Read the model definition and answer for the solid it produces. Units are mm, in the model's axes. A direction names the side the tool comes from. Give positions to 0.01 mm unless a question says otherwise; leave off trailing zeros. Order: outer loops, then holes, each group sorted by start corner. A loop starts at its lowest first (then second) coordinate and runs counter-clockwise, first axis right, second up. Notation, with made-up numbers: (20, -38.5) - (45, -38.5) arc R17 ccw to (45, -26.5) - close; hole circle Ø11 at (-33, 75.25). An arc over 180 degrees is marked (long way). Use a Markdown table: item, result. Add a question column.
1. For a pull along Z with two mould halves and no side action, classify faces 1 (the flat face through (33, 14, 40)), 2 (the cylindrical face through (124.91, 3.17, 0.9)), 3 (the flat face through (-2, 65, 22)), 4 (the cylindrical face through (-124.91, 3.17, 44.1)) as released by +Z, released by -Z, zero draft, split by the parting line, or undercut.
2. A cutting plane is placed at A-A on x = -21. Determine the outline of the cut face in (y, z).
3. Consider L1, parallel to Z at x = 17, y = -53; L2, parallel to Y at x = 48, z = 32; L3, parallel to X at y = 0, z = 3. Determine where each line is inside the solid, lowest interval first.
4. A cutting plane is placed at B-B on z = 31.5. Determine the outline of the cut face in (x, y).
5. A flat-ended cylindrical pin translates along its axis: P1, Ø17.5, axis at x = 11.5, z = 15, coming from the -Y side. Find the tip coordinate at first contact, or state that the pin passes through.
6. A cutting plane is placed at C-C on y = -21. State how many separate pieces and enclosed holes the cut face has, and give its area (3 significant figures).
7. Which of the six approach directions +Z, -Z, +X, -X, +Y, -Y give full straight-line access (tool end or side, diameter ignored) to faces 5 (the flat face through (-33, 18, 0)), 6 (the flat face through (33, 14, 5))?
Autodesk Inventor part; units mm, degrees
ref_plane "Work Plane2" through (142.5, 0, 0) normal (1, 0, 0) x (0, 1, 0)
ref_plane "Work Plane3" through (140, 0, 0) normal (1, 0, 0) x (0, 1, 0)
ref_plane "XZ Plane" through (0, 0, 0) normal (0, 1, 0) x (-1, 0, 0)
sketch "Sketch1" plane through (0, 0, 0) normal (0, 0, 1) x (1, 0, 0)
  circle A0 centre (0, 0) radius 35
  line L0 (0, 0) -> (0, 35)
  line L1 (0, 0) -> (0, -35)
  line L2 (110, -60) -> (141.25, 65)
  line L3 (-110, -60) -> (-141.25, 65)
  line L4 (0, -35) -> (0, -60)
  line L5 (0, -60) -> (110, -60)
  line L6 (0, -60) -> (-110, -60)
  line L7 (0, 35) -> (0, 65)
  line L8 (0, 65) -> (141.25, 65)
  line L9 (0, 65) -> (-141.25, 65)
extrude "Extrusion3" add sketch "Sketch1" along normal blind 45 contours A0 L7 L8 L2 L5 L4 | A0 L4 L6 L3 L9 L7
ref_plane "Work Plane2" through (142.5, 0, 0) normal (1, 0, 0) x (0, 1, 0)
fillet "Fillet2" radius 3 8 edges at (-141.25, 65, 22.5) (141.25, 65, 22.5) (125.625, 2.5, 45) (-125.625, 2.5, 45) (-125.625, 2.5, 0) (125.625, 2.5, 0) (0, -60, 0) (0, -60, 45)
sketch "Sketch5" plane through (142.5, 0, 0) normal (1, 0, 0) x (0, 1, 0)
  point P0 (0, 0)
ref_plane "Work Plane3" through (140, 0, 0) normal (1, 0, 0) x (0, 1, 0)
sketch "Sketch6" plane through (140, 0, 0) normal (1, 0, 0) x (0, 1, 0)
  line L0 (-56.5599, 40) -> (60, 40)
  line L1 (60, 40) -> (60, 5)
  line L2 (60, 5) -> (-60.1868, 5)
  line L3 (-56.5599, 40) -> (60, 5) construction
  line L4 (60, 40) -> (-60.1868, 5) construction
  line L5 (65, 0) -> (65, 45)
  line L6 (-56.5599, 40) -> (-64.3318, 40)
  line L7 (-64.3318, 40) -> (-64.3318, 5)
  line L8 (-64.3318, 5) -> (-60.1868, 5)
  line L9 (64.9104, 45) -> (-57, 45)
  line L10 (-57, 0) -> (64.9104, 0)
  point P0 (0, 0)
  point P1 (0.8272, 22.7681)
  dimension "d33" = 5
  dimension "d36" = 5
  dimension "d37" = 5
extrude "Extrusion5" cut sketch "Sketch6" against normal blind 1000
properties part number "sambungan leaf spring" material "Steel, Mild"
Output values:
| question | item | result |
|---|---|---|
| 1 | face 1 | undercut |
| 1 | face 2 | released by -Z |
| 1 | face 3 | zero draft |
| 1 | face 4 | released by +Z |
| 2 | outline | (-60, 3) arc R3 ccw to (-57, 0) - (-28, 0) - (-28, 5) - (-60, 5) - close; (-60, 40) - (-28, 40) - (-28, 45) - (-57, 45) arc R3 ccw to (-60, 42) - close; (28, 0) - (65, 0) - (65, 45) - (28, 45) - (28, 40) - (60, 40) - (60, 5) - (28, 5) - close |
| 3 | L1 | 0 to 5, 40 to 45 |
| 3 | L2 | 60 to 65 |
| 3 | L3 | -125 to -35, 35 to 125 |
| 4 | outline | (-140.32, 61.27) - (-140, 60) - (140, 60) - (140.32, 61.27) arc R3 ccw to (137.41, 65) - (-137.41, 65) arc R3 ccw to start |
| 5 | P1 | y = 60 |
| 6 | separate pieces | 4 |
| 6 | enclosed holes | 0 |
| 6 | area | 1,830 mm² |
| 7 | face 5 | -Z, +X, -X, +Y, -Y |
| 7 | face 6 | +X, -X, -Y |
